```python
from build123d import *

# Parameters (mm, degrees)
SKETCH1_R           = 2.4
BOSS_EXTRUDE1_DEPTH = 7.8
SKETCH2_R           = 3.05
CUT_EXTRUDE1_DEPTH  = 0.8
SKETCH3_R           = 3.05
CUT_EXTRUDE2_DEPTH  = 0.8


with BuildPart() as part:
    # Sketch1 → Boss-Extrude1 (new body)
    with BuildSketch(Plane(origin=(0, 0, 0), x_dir=(1, 0, 0), z_dir=(0, 1, 0))):
        with BuildLine():
            Line((-39.256074834, -14.981858177), (-26.182604436, -14.980554672))
            Line((-26.182604436, -14.980554672), (-26.185636373, 15.428181457))
            ThreePointArc((-26.185636373, 15.428181457), (-22.535634636, 19.078177837), (-18.885638256, 15.428176099))
            Line((-18.885638256, 15.428176099), (-18.882245203, -18.602359628))
            ThreePointArc((-18.882245203, -18.602359628), (-19.783925456, -21.035198794), (-22.073348778, -22.255966806))
            Line((-22.073348778, -22.255966806), (-38.897547418, -22.273048621))
            ThreePointArc((-38.897547418, -22.273048621), (-42.812314517, -18.811138133), (-39.256074834, -14.981858177))
        make_face()
        with Locations((-39.165637315, -18.631821222)):
            Circle(SKETCH1_R, mode=Mode.SUBTRACT)
        with Locations((-30.850637315, -18.631821222)):
            Circle(SKETCH1_R, mode=Mode.SUBTRACT)
        with Locations((-22.535637315, -18.631821222)):
            Circle(SKETCH1_R, mode=Mode.SUBTRACT)
        with Locations((-22.535637315, 15.428178778)):
            Circle(SKETCH1_R, mode=Mode.SUBTRACT)
        with Locations((-22.535637315, 6.913178778)):
            Circle(SKETCH1_R, mode=Mode.SUBTRACT)
        with Locations((-22.535637315, -1.601821222)):
            Circle(SKETCH1_R, mode=Mode.SUBTRACT)
        with Locations((-22.535637315, -10.116821222)):
            Circle(SKETCH1_R, mode=Mode.SUBTRACT)
    extrude(amount=BOSS_EXTRUDE1_DEPTH)

    # Sketch2 → Cut-Extrude1 (cut)
    with BuildSketch(Plane(origin=(0, 7.8, 0), x_dir=(1, 0, 0), z_dir=(0, 1, 0))):
        with Locations((-39.165637315, -18.631821222)):
            Circle(SKETCH2_R)
        with Locations((-30.850637315, -18.631821222)):
            Circle(SKETCH2_R)
        with Locations((-22.535637315, -18.631821222)):
            Circle(SKETCH2_R)
        with Locations((-22.535637315, -10.116821222)):
            Circle(SKETCH2_R)
        with Locations((-22.535637315, -1.601821222)):
            Circle(SKETCH2_R)
        with Locations((-22.535637315, 6.913178778)):
            Circle(SKETCH2_R)
        with Locations((-22.535637315, 15.428178778)):
            Circle(SKETCH2_R)
    extrude(amount=-CUT_EXTRUDE1_DEPTH, mode=Mode.SUBTRACT)

    # Sketch3 → Cut-Extrude2 (cut)
    with BuildSketch(Plane.XZ):
        with Locations((-30.850637315, 18.631821222)):
            Circle(SKETCH3_R)
        with Locations((-39.165637315, 18.631821222)):
            Circle(SKETCH3_R)
        with Locations((-22.535637315, 18.631821222)):
            Circle(SKETCH3_R)
        with Locations((-22.535637315, 10.116821222)):
            Circle(SKETCH3_R)
        with Locations((-22.535637315, 1.601821222)):
            Circle(SKETCH3_R)
        with Locations((-22.535637315, -6.913178778)):
            Circle(SKETCH3_R)
        with Locations((-22.535637315, -15.428178778)):
            Circle(SKETCH3_R)
    extrude(amount=-CUT_EXTRUDE2_DEPTH, mode=Mode.SUBTRACT)


solid = part.part
```
Work out the finished part from the listing and answer in its coordinate system (mm). A direction names the side the tool comes from. Round coordinates to 2 decimals unless told otherwise and drop trailing zeros. Write each loop counter-clockwise with the first axis right and the second up, starting at its lowest first coordinate (ties: lowest second). Pieces come first, ordered by that corner, then holes. Notation, with made-up numbers: (14.5, 16.5) -> (71.5, 16.5) arc R10 ccw to (71.5, 33.5) -> close; hole circle Ø4 at (87, 87). An arc over 180 degrees is marked (long way). Write each question's results on one line, items separated by ' | '.
Q1. Flat-ended cylindrical pins translate along their axes: P1, Ø5.5, axis at x = -22.54, z = 10.12, coming from the -Y side; P2, Ø2.5, axis at x = -32, y = 2.5, coming from the -Z side; P3, Ø2.5, axis at y = 2.5, z = 6, coming from the -X side. Find the tip coordinate at first contact, or state that the pin passes through.
Data:
P1: y = 0.8 | P2: z = 14.98 | P3: x = -26.18
Q2. Section D-D, the plane z = -11.5 is taken. Write down the section's boundary in (x, y).
Data:
outline: (-26.19, 0) -> (-18.89, 0) -> (-18.89, 7.8) -> (-26.19, 7.8) -> close
Q3. Straight lines are drawn through the part: line 1 along Z through (x, y) = (-22.75, 6.75); line 2 along Z through (x, y) = (-22.75, 0.5); line 3 along X through (y, z) = (1, 20). For each, find the intervals that lie inside material, in ascending order. Write a range as [from, to].
Data:
line 1: [-19.07, -17.82], [-13.04, -9.3], [-4.52, -0.79], [3.99, 7.73], [12.51, 16.24], [21.02, 22.26] | line 2: [-19.07, -18.47], [-12.39, -9.96], [-3.87, -1.44], [4.64, 7.07], [13.16, 15.59], [21.67, 22.26] | line 3: [-42.55, -41.14], [-37.19, -32.82], [-28.88, -24.51], [-20.56, -19.15]
Q4. Section C-C, the plane x = -29.25 is taken. Write down the section's boundary in (y, z), then the cut area to 3 significant figures.
Data:
outline: (0, 14.98) -> (7.8, 14.98) -> (7.8, 16.04) -> (7, 16.04) -> (7, 16.84) -> (0.8, 16.84) -> (0.8, 16.04) -> (0, 16.04) -> close; (0, 21.23) -> (0.8, 21.23) -> (0.8, 20.42) -> (7, 20.42) -> (7, 21.23) -> (7.8, 21.23) -> (7.8, 22.26) -> (0, 22.26) -> close | area: 26.3 mm^2
Q5. Section B-B, the plane y = 4.75 is taken. Write down the section's boundary in (x, z), then the cut area to 3 significant figures.
Data:
outline: (-39.26, 14.98) -> (-26.18, 14.98) -> (-26.19, -15.43) arc R3.65 ccw to (-18.89, -15.43) -> (-18.88, 18.6) arc R3.65 ccw to (-22.07, 22.26) -> (-38.9, 22.27) arc R3.65 ccw (long way) to start; hole circle Ø4.8 at (-39.17, 18.63); hole circle Ø4.8 at (-30.85, 18.63); hole circle Ø4.8 at (-22.54, -15.43); hole circle Ø4.8 at (-22.54, -6.91); hole circle Ø4.8 at (-22.54, 1.6); hole circle Ø4.8 at (-22.54, 10.12); hole circle Ø4.8 at (-22.54, 18.63) | area: 282 mm^2
Q6. Section A-A, the plane x = -38 is taken. Write down the section's boundary in (y, z), then the cut area to 3 significant figures.
Data:
outline: (0, 14.98) -> (7.8, 14.98) -> (7.8, 15.81) -> (7, 15.81) -> (7, 16.53) -> (0.8, 16.53) -> (0.8, 15.81) -> (0, 15.81) -> close; (0, 21.45) -> (0.8, 21.45) -> (0.8, 20.73) -> (7, 20.73) -> (7, 21.45) -> (7.8, 21.45) -> (7.8, 22.27) -> (0, 22.27) -> close | area: 21.8 mm^2
Q7. Which of the six approach directions +Z, -Z, +X, -X, +Y, -Y give full straight-line access (tool end or side, diameter ignored) to faces 1 (the cylindrical face through (-27.94, 7.41, 17.72)), 2 (the cylindrical face through (-37.875, 3.857, 16.608)), 3 (the cylindrical face through (-28.033, 0.394, 17.464))?
Data:
face 1: +Y | face 2: +Y, -Y | face 3: -Y
Q8. Determine the mould class of faces 4 (the cylindrical face through (-22.616, 3.845, -19.077)), 5 (the flat face through (-25, 7.8, 8)), 6 (the cylindrical face through (-28.56, 3.86, 17.91)), 7 (the cylindrical face through (-23.06, 3.86, -4.57)) for opening direction Z: released by +Z, released by -Z, zero draft, split by the parting line, or undercut.
Data:
face 4: released by -Z | face 5: zero draft | face 6: undercut | face 7: undercut
